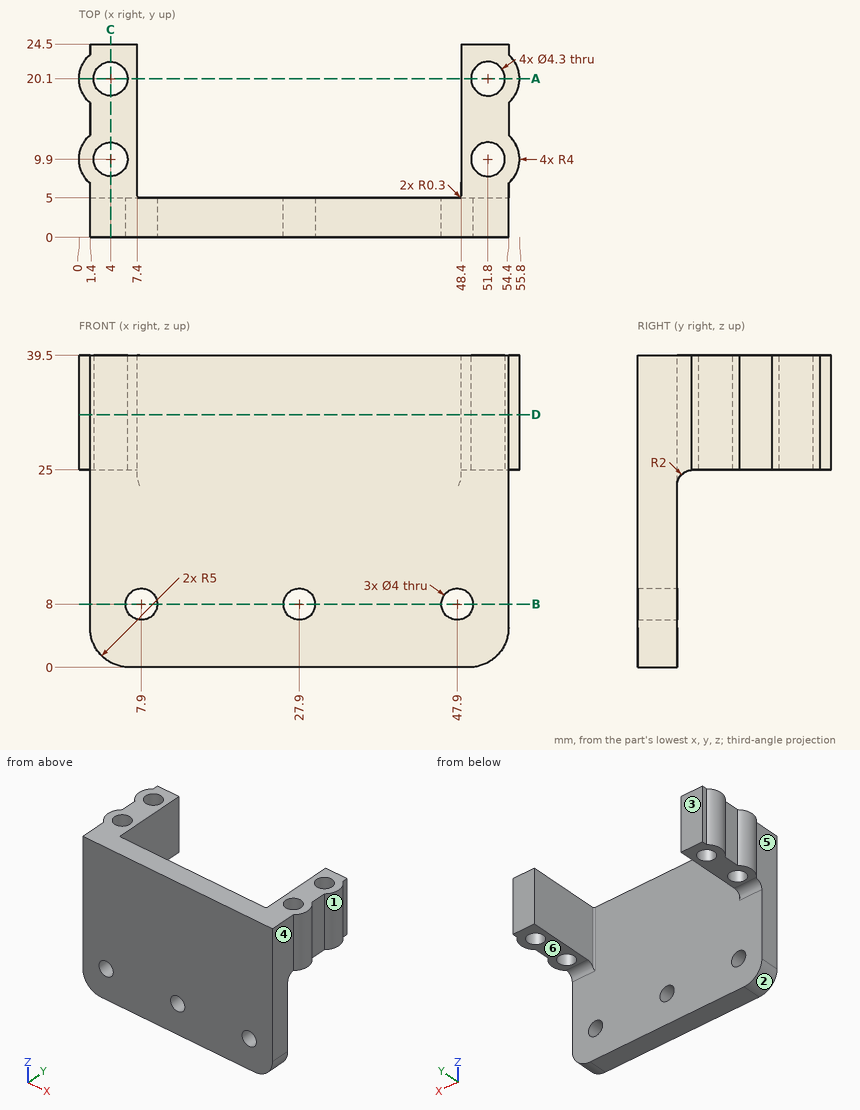
Geometry check sheet. Reference: drawing and pictorial views, mm from the part's lowest x, y, z. A direction names the side the tool comes from. Give positions to 0.01 mm unless a question says otherwise; leave off trailing zeros. Write each loop counter-clockwise with the first axis right and the second up, starting at its lowest first coordinate (ties: lowest second). Pieces come first, ordered by that corner, then holes.
Item 1: Access from +Z, -Z, +X, -X, +Y, -Y to the whole of each face (thin tool, end or side, straight path). Record for the marked faces 4, 5 and 6.
Item 2: Cross-section at D-D (z = 32). Enter the section's corners in (x, y).
Item 3: Scan lines: L1, parallel to X at y = 3.2, z = 8; L2, parallel to X at y = 15.5, z = 31; L3, parallel to Z at x = 47.9, y = 1.35. Record each from-to range of solid material in increasing order.
Item 4: Cross-section at C-C (x = 4). Enter the section's corners in (y, z), and give its area (3 significant figures).
Item 5: Cross-section at B-B (z = 8). Enter the section's corners in (x, y), and give its area (3 significant figures).
Item 6: Draft check along Y on the marked faces 1, 2 and 3. Enter one of: released by +Y, released by -Y, zero draft, split by the parting line, or undercut.
Item 7: Cross-section at A-A (y = 20.1). Enter the section's corners in (x, z).
Item 8: Gauge pin test, flat ends, axial feed: pin 1 (8 mm diameter, centred on x = 51.5, y = 16, fed in from -Z); pin 2 (6 mm diameter, centred on x = 10, z = 17, fed in from +Y); pin 3 (5.5 mm diameter, centred on y = 4, z = 30, fed in from +X). Record the tip position at first contact, or that the pin passes through.
Report:
1. face 4: +Z, -Z, +X, -Y
1. face 5: +Z, -Z, -X, -Y
1. face 6: -Z, +X, -X, +Y
2. outline: (1.4, 0) - (54.4, 0) - (54.4, 6.86) arc R4 ccw to (54.4, 12.94) - (54.4, 17.06) arc R4 ccw to (54.4, 23.14) - (54.4, 24.5) - (48.4, 24.5) - (48.4, 5.3) arc R0.3 cw to (48.1, 5) - (7.7, 5) arc R0.3 cw to (7.4, 5.3) - (7.4, 24.5) - (1.4, 24.5) - (1.4, 23.14) arc R4 ccw to (1.4, 17.06) - (1.4, 12.94) arc R4 ccw to (1.4, 6.86) - close; hole circle Ø4.3 at (4, 9.9); hole circle Ø4.3 at (4, 20.1); hole circle Ø4.3 at (51.8, 9.9); hole circle Ø4.3 at (51.8, 20.1)
3. L1: x = 1.4 to 5.9, 9.9 to 25.9, 29.9 to 45.9, 49.9 to 54.4
3. L2: x = 1.4 to 7.4, 48.4 to 54.4
3. L3: z = 0 to 6, 10 to 39.5
4. outline: (0, 0.61) - (5, 0.61) - (5, 23) arc R2 cw to (7, 25) - (7.75, 25) - (7.75, 39.5) - (0, 39.5) - close; (12.05, 25) - (17.95, 25) - (17.95, 39.5) - (12.05, 39.5) - close; (22.25, 25) - (24.5, 25) - (24.5, 39.5) - (22.25, 39.5) - close
4. area: 353 mm2
5. outline: (1.4, 0) - (5.9, 0) - (5.9, 5) - (1.4, 5) - close; (9.9, 0) - (25.9, 0) - (25.9, 5) - (9.9, 5) - close; (29.9, 0) - (45.9, 0) - (45.9, 5) - (29.9, 5) - close; (49.9, 0) - (54.4, 0) - (54.4, 5) - (49.9, 5) - close
5. area: 205 mm2
6. face 1: undercut
6. face 2: zero draft
6. face 3: released by +Y
7. outline: (0, 25) - (1.85, 25) - (1.85, 39.5) - (0, 39.5) - close; (6.15, 25) - (7.4, 25) - (7.4, 39.5) - (6.15, 39.5) - close; (48.4, 25) - (49.65, 25) - (49.65, 39.5) - (48.4, 39.5) - close; (53.95, 25) - (55.8, 25) - (55.8, 39.5) - (53.95, 39.5) - close
8. pin 1: stops at z = 25
8. pin 2: stops at y = 5
8. pin 3: stops at x = 54.4
